Source: CAD feature listing. Evaluate the final solid. Frame: model axes, mm. Give positions to 0.01 mm unless a question says otherwise; leave off trailing zeros. Order: outer loops, then holes, each group sorted by start corner. A loop starts at its lowest first (then second) coordinate and runs counter-clockwise, first axis right, second up. Notation, with made-up numbers: (39.25, -10) -> (43.25, -10) arc R28 cw to (43.25, 16) -> close; hole circle Ø8 at (-25.5, 6.25). An arc over 180 degrees is marked (long way). Use one line per item in the form item = value. Start each with the question number.
from build123d import *

# Parameters (mm, degrees)
SKETCH2_W           = 40
SKETCH2_H           = 225
BOSS_EXTRUDE1_DEPTH = 4
SKETCH3_R           = 2
CUT_EXTRUDE1_DEPTH  = 115.333940718
LPATTERN1_COUNT     = 7
LPATTERN1_PITCH     = 10
FILLET2_R           = 20


with BuildPart() as part:
    # Sketch2 → Boss-Extrude1 (new body)
    with BuildSketch(Plane.XY):
        Rectangle(SKETCH2_W, SKETCH2_H)
    extrude(amount=BOSS_EXTRUDE1_DEPTH)

    # Sketch3 → Cut-Extrude1 (cut, through all)
    with BuildSketch(Plane.XY.offset(4)):
        with Locations((-10, -100)):
            Circle(SKETCH3_R)
        with Locations((10, -100)):
            Circle(SKETCH3_R)
    cut_extrude1 = extrude(amount=-CUT_EXTRUDE1_DEPTH, mode=Mode.SUBTRACT)

    # LPattern1: Cut-Extrude1 ×7
    with Locations(*[(0, i * LPATTERN1_PITCH, 0) for i in range(1, LPATTERN1_COUNT)]):
        add(cut_extrude1, mode=Mode.SUBTRACT)

    # Fillet2
    fillet2_edges = [part.edges().sort_by_distance(p)[0] for p in [
        (20, -112.5, 2),
        (-20, -112.5, 2),
    ]]
    fillet(fillet2_edges, radius=FILLET2_R - 0.0001)  # a hair under: the kernel refuses the full size


solid = part.part
1) Cut plane D-D, the plane y = -100. Return the cut outline in (x, z), plus the area to 3 significant figures.
2) Pin query (flat end, axial travel): pin 1 (1.5 mm diameter, centred on x = -13.5, y = -75, fed in from -Z); pin 2 (1.5 mm diameter, centred on x = -4.5, z = 2, fed in from -Y). Return the tip coordinate at first contact, or that it passes through.
3) Material intervals for probe 1 along Y at (x, z) = (-14, 2.45); probe 2 along Y at (x, z) = (-13, 3.5), sorted ascending.
4) Cut plane B-B, the plane y = -40. Return the cut outline in (x, z).
5) Cut plane A-A, the plane z = 3.2. Count the separate pieces of the cut face and the enclosed holes in it, plus the area to 3 significant figures.
6) Draft query along Y for faces 1 (the face through (10, -78, 2)), 2 (the face through (-10, -88, 2)), 3 (the face through (-20, 9, 2)), 4 (the face through (0, 112.5, 2)). Return one class per face: +Y half, -Y half, draft (parallel to the pull), parting line (faces both ways), or undercut.
Output values:
q1.outline = (-18.54, 0) -> (-12, 0) -> (-12, 4) -> (-18.54, 4) -> close; (-8, 0) -> (8, 0) -> (8, 4) -> (-8, 4) -> close; (12, 0) -> (18.54, 0) -> (18.54, 4) -> (12, 4) -> close
q1.area = 116 mm^2
q2.pin_1 = 0
q2.pin_2 = -112.15
q3.probe_1 = -106.78 to 112.5
q3.probe_2 = -107.7 to 112.5
q4.outline = (-20, 0) -> (-12, 0) -> (-12, 4) -> (-20, 4) -> close; (-8, 0) -> (8, 0) -> (8, 4) -> (-8, 4) -> close; (12, 0) -> (20, 0) -> (20, 4) -> (12, 4) -> close
q5.separate_pieces = 1
q5.enclosed_holes = 14
q5.area = 8,650 mm^2
q6.face_1 = undercut
q6.face_2 = undercut
q6.face_3 = draft
q6.face_4 = +Y half
